The listing builds one solid part. Answer for the finished solid, in the listing's coordinates (mm). Round coordinates to 2 decimals unless told otherwise and drop trailing zeros. Loops run counter-clockwise (first coordinate to the right, second up) from the corner with the lowest first, then second, coordinate; pieces in that order, holes last. Notation, with made-up numbers: (33, 31.5) - (56, 31.5) arc R28 ccw to (56, 60.5) - close; hole circle Ø8 at (-16, -35). An arc over 180 degrees is marked (long way). One line per item, written item: value.
Autodesk Inventor part; units mm, degrees
ref_plane "YZ Plane" through (0, 0, 0) normal (1, 0, 0) x (0, 1, 0)
ref_plane "XZ Plane" through (0, 0, 0) normal (0, 1, 0) x (-1, 0, 0)
ref_plane "XY Plane" through (0, 0, 0) normal (0, 0, 1) x (1, 0, 0)
sketch "Sketch1" plane through (0, 0, 0) normal (0, 1, 0) x (-1, 0, 0)
  line L0 (0, 0) -> (165.1, 0)
  line L1 (177.8, 12.7) -> (177.8, 20.6375)
  line L2 (177.8, 20.6375) -> (0, 20.6375)
  line L3 (0, 20.6375) -> (0, 0)
  line L4 (165.1, 0) -> (177.8, 12.7)
  circle A0 centre (139.7, 7.9375) radius 3.3734
  circle A1 centre (63.5, 7.9375) radius 3.3734
  circle A2 centre (12.7, 7.9375) radius 3.3734
  point P0 (177.8, 0)
  dimension "d0" = 177.8
  dimension "d1" = 20.6375
  dimension "d2" = 12.7
  dimension "d3" = 12.7
  dimension "d4" = 12.7
  dimension "d5" = 12.7
  dimension "d6" = 12.7
  dimension "d7" = 12.7
  dimension "d8" = 63.5
  dimension "d9" = 139.7
  dimension "d10" = 6.7469
  dimension "d11" = 6.7469
  dimension "d12" = 6.7469
extrude "Extrusion1" add sketch "Sketch1" along normal blind 6.35
properties part number "gusset guard" material "Aluminum 6061"
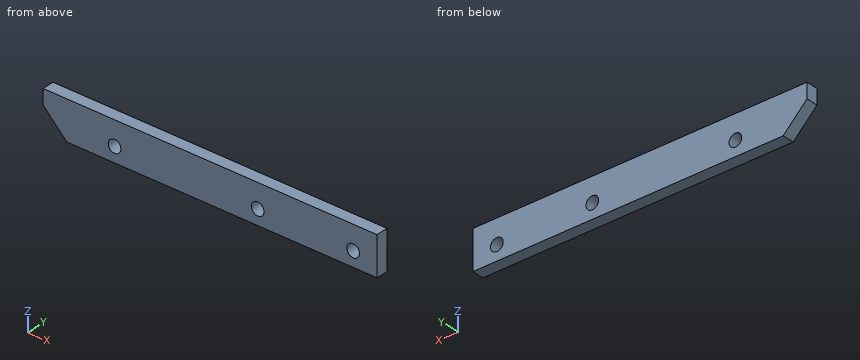
1) This flat-tipped pin is pushed along its axis until it touches: pin 1 Ø3 at (y, z) = (3.5, 9.5) entering from -X. Where does it stop, or does it pass through?
Final values:
pin 1: x = -176.1
2) Consider L1, parallel to Z at x = -63.5, y = 3.25; L2, parallel to X at y = 1.5, z = 6.5; L3, parallel to X at y = 5, z = 10.25. Determine where each line is inside the solid, lowest interval first.
Final values:
L1: 0 to 4.56, 11.31 to 20.64
L2: -171.6 to -142.75, -136.65 to -66.55, -60.45 to -15.75, -9.65 to 0
L3: -175.35 to -142.16, -137.24 to -65.96, -61.04 to -15.16, -10.24 to 0
3) A cutting plane is placed at A-A on x = -12.7. Give the vertices of the cut face in (y, z), and give its area (3 significant figures).
Final values:
outline: (0, 0) - (6.35, 0) - (6.35, 4.56) - (0, 4.56) - close; (0, 11.31) - (6.35, 11.31) - (6.35, 20.64) - (0, 20.64) - close
area: 88.2 mm2
4) A cutting plane is placed at B-B on y = 3. Give the vertices of the cut face in (x, z).
Final values:
outline: (-177.8, 12.7) - (-165.1, 0) - (0, 0) - (0, 20.64) - (-177.8, 20.64) - close; hole circle Ø6.75 at (-139.7, 7.94); hole circle Ø6.75 at (-63.5, 7.94); hole circle Ø6.75 at (-12.7, 7.94)
